from build123d import *

# Parameters (mm, degrees)
F1_DEPTH = 82.55
F2_R     = 17.4625
F3_DEPTH = 25.401
F4_R     = 17.4625
F5_DEPTH = 12.701


with BuildPart() as f1:
    # F0 (on Front) → F1 (new body)
    with BuildSketch(Plane.XZ):
        Polygon((0, 127), (0, 0), (190.5, 0), (190.5, 12.7), (25.4, 12.7), (25.4, 127), align=None)
    extrude(amount=F1_DEPTH)

    # F2 (on face) → F3 (cut, through all)
    with BuildSketch(Plane.YZ.offset(25.4)):
        with Locations((-41.275, 69.85)):
            Circle(F2_R)
        with BuildLine():
            ThreePointArc((-82.55, 69.85), (-41.275, 111.125), (0, 69.85))
            Line((0, 69.85), (0, 127))
            Line((0, 127), (-82.55, 127))
            Line((-82.55, 127), (-82.55, 69.85))
        make_face()
    extrude(amount=-F3_DEPTH, mode=Mode.SUBTRACT)

    # F4 (on face) → F5 (cut, through all)
    with BuildSketch(Plane.XY.offset(12.7)):
        with Locations((152.4, -41.275)):
            Circle(F4_R)
        with Locations((76.2, -41.275)):
            Circle(F4_R)
    extrude(amount=-F5_DEPTH, mode=Mode.SUBTRACT)


solid = f1.part
Design review of the part built by this model. Coordinates are the model's own, in mm. A direction names the side the tool comes from. Give positions to 0.01 mm unless a question says otherwise; leave off trailing zeros. Loops run counter-clockwise (first coordinate to the right, second up) from the corner with the lowest first, then second, coordinate; pieces in that order, holes last. Notation, with made-up numbers: (15, -21) - (39, -21) arc R29 cw to (39, 5) - close; hole circle Ø4 at (49.5, 2.5). An arc over 180 degrees is marked (long way). Use CSV: the item, a comma, the result in double quotes. Start each with the question number.
1. Insertion check: P1, Ø25, axis at x = 104.5, y = -54.5, coming from the +Z side; P2, Ø21, axis at y = -41.275, z = 69.85, coming from the +X side. Each pin has a flat end and moves straight along its axis. Give the tip position at first contact, or say it passes through.
2. Add section C-C (y = -28.5). State the section outline as (x, z) points, plus the area to 3 significant figures.
3. Machinability: for faces 4 (the flat face through (25.4, -41, 50)), 5 (the cylindrical face through (12.9, -54.1, 81.7)), which of the approach directions +Z, -Z, +X, -X, +Y, -Y give a long, thin tool a straight path to every point of the face, cutting with its end or side? Answer none if there is none.
4. Add section B-B (z = 84). State the section outline as (x, y) points.
5. Add section A-A (x = 152.4). State the section outline as (y, z) points, plus the area to 3 significant figures.
6. Wall thickness on L1, parallel to Y at x = 152.4, z = 6; L2, parallel to Z at x = 44, y = -48; L3, parallel to X at y = -59, z = 84.5: over which ranges is each line inside the solid? List them lowest first.
7. Add section D-D (y = -11). State the section outline as (x, z) points, plus the area to 3 significant figures.
8. Draft analysis for pull direction Y (two halves, no side actions). For faces 1 (the flat face through (60, -82.55, 12)), 2 (the flat face through (94, -41, 0)), 3 (the cylindrical face through (92.331, -47.963, 6.439)), state which applies: released by +Y, released by -Y, zero draft, split by the parting line, or undercut.
Results found:
1,P1,"stops at z = 12.7"
1,P2,"passes through"
2,outline,"(0, 0) - (64.29, 0) - (64.29, 12.7) - (25.4, 12.7) - (25.4, 57.94) - (0, 57.94) - close; (0, 81.76) - (25.4, 81.76) - (25.4, 109.1) - (0, 109.1) - close; (88.11, 0) - (140.49, 0) - (140.49, 12.7) - (88.11, 12.7) - close; (164.31, 0) - (190.5, 0) - (190.5, 12.7) - (164.31, 12.7) - close"
2,area,"3,660 mm²"
3,face 4,"+Z, +X, +Y, -Y"
3,face 5,"+X, -X"
4,outline,"(0, -80.05) - (25.4, -80.05) - (25.4, -51.51) - (0, -51.51) - close; (0, -31.04) - (25.4, -31.04) - (25.4, -2.5) - (0, -2.5) - close"
5,outline,"(-82.55, 0) - (-58.74, 0) - (-58.74, 12.7) - (-82.55, 12.7) - close; (-23.81, 0) - (0, 0) - (0, 12.7) - (-23.81, 12.7) - close"
5,area,"605 mm²"
6,L1,"y = -82.55 to -58.74, -23.81 to 0"
6,L2,"z = 0 to 12.7"
6,L3,"x = 0 to 25.4"
7,outline,"(0, 0) - (190.5, 0) - (190.5, 12.7) - (25.4, 12.7) - (25.4, 97.9) - (0, 97.9) - close"
7,area,"4,580 mm²"
8,face 1,"released by -Y"
8,face 2,"zero draft"
8,face 3,"undercut"
